from build123d import *

# Parameters (mm, degrees)
SKETCH1_W           = 139.192
SKETCH1_H           = 177.292
BOSS_EXTRUDE1_DEPTH = 6.35
SKETCH2_W           = 6.55
SKETCH2_H           = 177.292
CUT_EXTRUDE1_DEPTH  = 3.375
SKETCH3_W           = 12.7
SKETCH3_H           = 12.7
BOSS_EXTRUDE2_DEPTH = 6.35
FILLET1_R           = 6.35
SKETCH4_R           = 3.175
CUT_EXTRUDE2_DEPTH  = 236.609200644
SKETCH5_R           = 2.286
CUT_EXTRUDE3_DEPTH  = 12.7


with BuildPart() as part:
    # Sketch1 → Boss-Extrude1 (new body)
    with BuildSketch(Plane(origin=(0, 0, 0), x_dir=(1, 0, 0), z_dir=(0, 1, 0))):
        with Locations((69.596, 88.646)):
            Rectangle(SKETCH1_W, SKETCH1_H)
    extrude(amount=BOSS_EXTRUDE1_DEPTH)

    # Sketch2 → Cut-Extrude1 (cut)
    with BuildSketch(Plane(origin=(0, 6.35, 0), x_dir=(1, 0, 0), z_dir=(0, 1, 0))):
        with Locations((135.917, 88.646)):
            Rectangle(SKETCH2_W, SKETCH2_H)
        with Locations((3.275, 88.646)):
            Rectangle(SKETCH2_W, SKETCH2_H)
    extrude(amount=-CUT_EXTRUDE1_DEPTH, mode=Mode.SUBTRACT)

    # Sketch3 → Boss-Extrude2 (add)
    with BuildSketch(Plane(origin=(0, 6.35, 0), x_dir=(1, 0, 0), z_dir=(0, 1, 0))):
        with Locations((69.596, 183.642)):
            Rectangle(SKETCH3_W, SKETCH3_H)
    extrude(amount=-BOSS_EXTRUDE2_DEPTH)

    # Fillet1
    fillet1_edges = [part.edges().sort_by_distance(p)[0] for p in [
        (63.246, 3.175, -189.992),
        (75.946, 3.175, -189.992),
    ]]
    fillet(fillet1_edges, radius=FILLET1_R - 0.0001)  # a hair under: the kernel refuses the full size

    # Sketch4 → Cut-Extrude2 (cut, through all)
    with BuildSketch(Plane(origin=(0, 6.35, 0), x_dir=(1, 0, 0), z_dir=(0, 1, 0))):
        with Locations(Location((69.596, 183.642, 0), (0, 0, 270))):
            Circle(SKETCH4_R)
    extrude(amount=-CUT_EXTRUDE2_DEPTH, mode=Mode.SUBTRACT)

    # Sketch5 → Cut-Extrude3 (cut)
    with BuildSketch(Plane.XZ):
        with Locations(Location((107.188, -10.414, 0), (0, 0, 270))):
            Circle(SKETCH5_R)
        with Locations(Location((97.282, -10.414, 0), (0, 0, 270))):
            Circle(SKETCH5_R)
        with Locations(Location((41.91, -10.414, 0), (0, 0, 270))):
            Circle(SKETCH5_R)
        with Locations(Location((32.004, -10.414, 0), (0, 0, 270))):
            Circle(SKETCH5_R)
    extrude(amount=-CUT_EXTRUDE3_DEPTH, mode=Mode.SUBTRACT)


solid = part.part
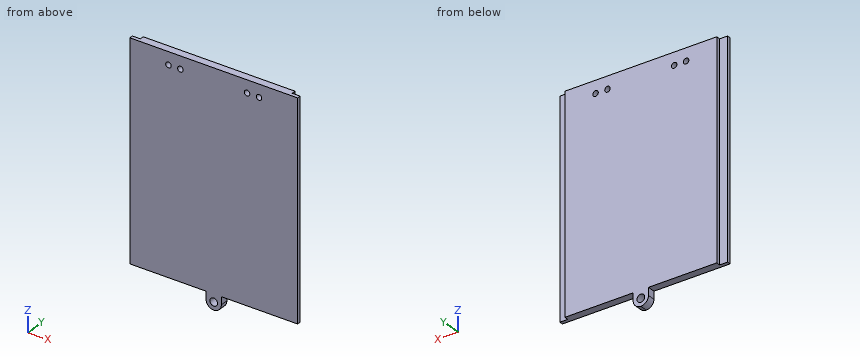
Source: CAD feature listing. Evaluate the final solid. Frame: model axes, mm. Give positions to 0.01 mm unless a question says otherwise; leave off trailing zeros. Order: outer loops, then holes, each group sorted by start corner. A loop starts at its lowest first (then second) coordinate and runs counter-clockwise, first axis right, second up. Notation, with made-up numbers: (64.25, 57.5) -> (87.25, 57.5) arc R30 cw to (87.25, 94.5) -> close; hole circle Ø3 at (-27.75, 39). An arc over 180 degrees is marked (long way). Use a Markdown table: item, result.
1) Ray query, line 1 along X through (y, z) = (2.5, -11); line 2 along X through (y, z) = (4.5, -48.5); line 3 along Z through (x, y) = (119, 5.75). Return the intervals inside material, ascending. Write a range as [from, to].
Answer list:
| item | result |
|---|---|
| line 1 | [0, 29.79], [34.21, 39.7], [44.12, 95.07], [99.49, 104.98], [109.4, 139.19] |
| line 2 | [6.55, 132.64] |
| line 3 | [-177.29, 0] |
2) Section query C-C, the plane z = -107.5. Return the cut outline in (x, y) (3 decimals), then the cut area to 3 significant figures.
Answer list:
| item | result |
|---|---|
| outline | (0, 0) -> (139.192, 0) -> (139.192, 2.975) -> (132.642, 2.975) -> (132.642, 6.35) -> (6.55, 6.35) -> (6.55, 2.975) -> (0, 2.975) -> close |
| area | 840 mm² |
3) Contact query for flat-ended pins moving along their axis: P1, Ø3.5, axis at x = 134.5, z = -93, coming from the +Y side (3 decimals); P2, Ø1.9, axis at x = 22.5, y = 2, coming from the -Z side; P3, Ø3, axis at y = 1.5, z = -180, coming from the -X side; P4, Ø5.5, axis at x = 69.596, z = -183.642, coming from the -Y side. Output: stop coordinate, or through.
Answer list:
| item | result |
|---|---|
| P1 | y = 2.975 |
| P2 | z = -177.29 |
| P3 | x = 63.25 |
| P4 | through |
4) Section query A-A, the plane x = 41.91. Return the cut outline in (y, z).
Answer list:
| item | result |
|---|---|
| outline | (0, -177.29) -> (6.35, -177.29) -> (6.35, -12.7) -> (0, -12.7) -> close; (0, -8.13) -> (6.35, -8.13) -> (6.35, 0) -> (0, 0) -> close |
5) Section query D-D, the plane x = 114.5. Return the cut outline in (y, z), then the cut area to 3 significant figures.
Answer list:
| item | result |
|---|---|
| outline | (0, -177.29) -> (6.35, -177.29) -> (6.35, 0) -> (0, 0) -> close |
| area | 1,130 mm² |
6) Section query B-B, the plane y = 1.25. Count the separate pieces of the cut face and the enclosed holes in it, then the cut area to 3 significant figures.
Answer list:
| item | result |
|---|---|
| separate pieces | 1 |
| enclosed holes | 5 |
| area | 24,700 mm² |
